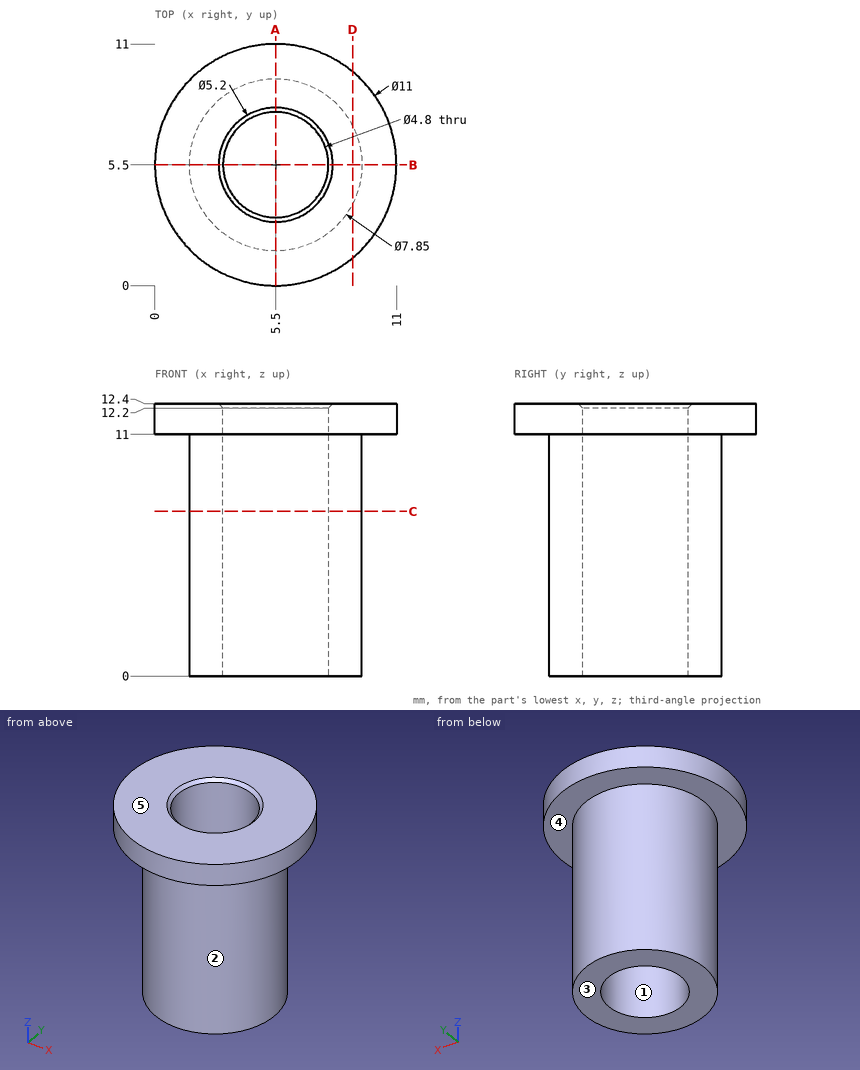
For this review, use the dimensioned drawing (mm, ordinates from the lowest corner) and the shaded views. A direction names the side the tool comes from. Give positions to 0.01 mm unless a question says otherwise; leave off trailing zeros. Loops run counter-clockwise (first coordinate to the right, second up) from the corner with the lowest first, then second, coordinate; pieces in that order, holes last.
Item 1: Tool access review of the marked faces 4 and 5: name each direction out of +Z, -Z, +X, -X, +Y, -Y from which nothing blocks a thin tool from reaching the whole face with its end or side.
Item 2: Draft analysis for pull direction Y (two halves, no side actions). For the marked faces 1, 2 and 3, state which applies: +Y half, -Y half, draft (parallel to the pull), parting line (faces both ways), or undercut.
Item 3: Take a section at D-D, the plane x = 9. State the section outline as (y, z) points, and give its area (3 significant figures).
Item 4: For line 1 along Y through (x, z) = (5.5, 3.5) (3 decimals); line 2 along Z through (x, y) = (6.75, 1.5); line 3 along Y through (x, z) = (6, 6.5), list the stretches that pass through material, from the lowest coordinate up.
Item 5: Take a section at C-C, the plane z = 7.5. State the section outline as (x, y) points (3 decimals).
Item 6: Take a section at A-A, the plane x = 5.5. State the section outline as (y, z) points (3 decimals), and give its area (3 significant figures).
Calculated:
1. face 4: -Z
1. face 5: +Z, +X, -X, +Y, -Y
2. face 1: undercut
2. face 2: parting line
2. face 3: draft
3. outline: (1.26, 11) - (3.72, 11) - (3.72, 0) - (7.28, 0) - (7.28, 11) - (9.74, 11) - (9.74, 12.4) - (1.26, 12.4) - close
3. area: 51.0 mm2
4. line 1: y = 1.575 to 3.1, 7.9 to 9.425
4. line 2: z = 11 to 12.4
4. line 3: y = 1.61 to 3.15, 7.85 to 9.39
5. outline: circle Ø7.85 at (5.5, 5.5); hole circle Ø4.8 at (5.5, 5.5)
6. outline: (0, 11) - (1.575, 11) - (1.575, 0) - (3.1, 0) - (3.1, 12.2) - (2.9, 12.4) - (0, 12.4) - close; (7.9, 0) - (9.425, 0) - (9.425, 11) - (11, 11) - (11, 12.4) - (8.1, 12.4) - (7.9, 12.2) - close
6. area: 42.2 mm2
